Geometry: see drawing. Coordinates: mm, zero at the bounding-box minimum. A direction names the side the tool comes from. Give positions to 0.01 mm unless a question says otherwise; leave off trailing zeros. Loops run counter-clockwise (first coordinate to the right, second up) from the corner with the lowest first, then second, coordinate; pieces in that order, holes last. Notation, with made-up numbers: M -11.5,60.25 L -1.5,60.25 A17 cw -1.5,81.25 Z; hole C 40.25,42.25 d11. An arc over 180 degrees is marked long. Put each result on its own line as item: value.
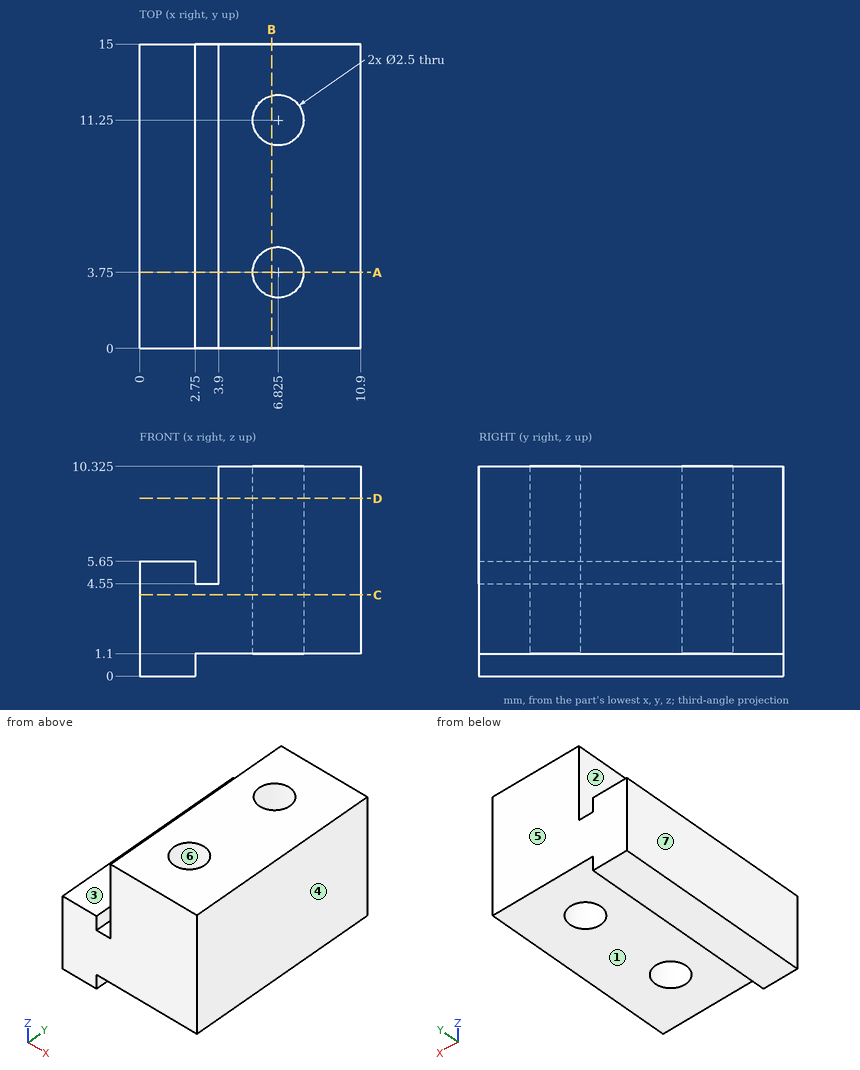
Item 1: Section B-B on x = 6.5. Output: boundary loops of the cut face in (y, z) (3 decimals).
Output values:
outline: M 0,1.1 L 2.543,1.1 L 2.543,10.325 L 0,10.325 Z; M 4.957,1.1 L 10.043,1.1 L 10.043,10.325 L 4.957,10.325 Z; M 12.457,1.1 L 15,1.1 L 15,10.325 L 12.457,10.325 Z
Item 2: Mould query, pull axis X, two halves, no side actions, for the marked faces 4, 5, 6 and 7. Classes: pulls with the +X half, pulls with the -X half, needs draft (parallel to the pull), parting line crosses it, or undercut.
Output values:
face 4: pulls with the +X half
face 5: needs draft
face 6: undercut
face 7: pulls with the -X half
Item 3: Pin query (flat end, axial travel): pin 1 Ø5 at (x, y) = (8.5, 3) entering from -Z; pin 2 Ø3 at (x, y) = (1.5, 9.5) entering from +Z; pin 3 Ø2 at (x, y) = (6.825, 11.25) entering from -Z. Return the tip coordinate at first contact, or that it passes through.
Output values:
pin 1: z = 1.1
pin 2: z = 5.65
pin 3: through
Item 4: Set-up query: the marked faces 1, 2 and 3. Return all of +Z, -Z, +X, -X, +Y, -Y with unobstructed straight access to the full face (end or side cutting, diameter ignored); none if empty.
Output values:
face 1: -Z, +X, +Y, -Y
face 2: +Z, +Y, -Y
face 3: +Z, -X, +Y, -Y
Item 5: Section D-D on z = 8.75. Output: boundary loops of the cut face in (x, y) (3 decimals), then the cut area to 3 significant figures.
Output values:
outline: M 3.9,0 L 10.9,0 L 10.9,15 L 3.9,15 Z; hole C 6.825,3.75 d2.5; hole C 6.825,11.25 d2.5
area: 95.2 mm²
Item 6: Section A-A on y = 3.75. Output: boundary loops of the cut face in (x, z) (3 decimals).
Output values:
outline: M 0,0 L 2.75,0 L 2.75,1.1 L 5.575,1.1 L 5.575,10.325 L 3.9,10.325 L 3.9,4.55 L 2.75,4.55 L 2.75,5.65 L 0,5.65 Z; M 8.075,1.1 L 10.9,1.1 L 10.9,10.325 L 8.075,10.325 Z
Item 7: Line query: probe 1 along Y at (x, z) = (7.75, 3); probe 2 along X at (y, z) = (8.75, 7); probe 3 along Z at (x, y) = (9.25, 11) (3 decimals). Output: solid intervals per line, ascending. Write a range as [from, to].
Output values:
probe 1: [0, 2.91], [4.59, 10.41], [12.09, 15]
probe 2: [3.9, 10.9]
probe 3: [1.1, 10.325]
Item 8: Section C-C on z = 4. Output: boundary loops of the cut face in (x, y) (3 decimals).
Output values:
outline: M 0,0 L 10.9,0 L 10.9,15 L 0,15 Z; hole C 6.825,3.75 d2.5; hole C 6.825,11.25 d2.5
